The model under review builds one solid part; all positions refer to its coordinate system, in mm. A direction names the side the tool comes from. Round coordinates to 2 decimals unless told otherwise and drop trailing zeros. Order: outer loops, then holes, each group sorted by start corner. A loop starts at its lowest first (then second) coordinate and runs counter-clockwise, first axis right, second up. Notation, with made-up numbers: M 75.5,73 L 132.5,73 A25 cw 132.5,96 Z; hole C 1,56 d5. An arc over 180 degrees is marked long. Answer as CSV lines item,"result". Start each with the question number.
from build123d import *

# Parameters (mm, degrees)
SKETCH_1_W             = 45
SKETCH_1_H             = 38.5
EXTRUDE_1_DEPTH        = 60
SKETCH_2_R             = 15.1
CUT_EXTRUDE_1_DEPTH    = 50
SKETCH_3_R             = 2.5
EXTRUDE_2_DEPTH        = 5
SKETCH_4_R             = 1.5
CUT_EXTRUDE_2_DEPTH    = 78.620873481
PATTERN_LINEAR_1_COUNT = 2
PATTERN_LINEAR_1_PITCH = 20
FILLET_1_R             = 10


with BuildPart() as part:
    # 草圖1 → 填料-伸長1 (new body)
    with BuildSketch(Plane(origin=(0, 0, 0), x_dir=(1, 0, 0), z_dir=(0, 1, 0))):
        with Locations((-2.5, 0.75)):
            Rectangle(SKETCH_1_W, SKETCH_1_H)
    extrude(amount=EXTRUDE_1_DEPTH)

    # 草圖2 → 除料-伸長1 (cut)
    with BuildSketch(Plane(origin=(0, 60, 0), x_dir=(1, 0, 0), z_dir=(0, 1, 0))):
        with Locations(Location((0, 0, 0), (0, 0, 270))):
            Circle(SKETCH_2_R)
    extrude(amount=-CUT_EXTRUDE_1_DEPTH, mode=Mode.SUBTRACT)

    # 草圖3 → 填料-伸長2 (add)
    with BuildSketch(Plane.XY.offset(18.5)):
        Polygon((-25, 0), (-25, -15.5), (-5, -15.5), (20, 0), align=None)
        with Locations((-17.5, -8)):
            Circle(SKETCH_3_R, mode=Mode.SUBTRACT)
    extrude(amount=-EXTRUDE_2_DEPTH)

    # 草圖4 → 除料-伸長2 (cut, through all)
    with BuildSketch(Plane(origin=(20, 0, 0), x_dir=(0, 0, -1), z_dir=(1, 0, 0))):
        with Locations((0, 20)):
            Circle(SKETCH_4_R)
    cut_extrude_2 = extrude(amount=-CUT_EXTRUDE_2_DEPTH, mode=Mode.SUBTRACT)

    # 直線複製排列1: 除料-伸長2 ×2
    with Locations(*[(0, i * PATTERN_LINEAR_1_PITCH, 0) for i in range(1, PATTERN_LINEAR_1_COUNT)]):
        add(cut_extrude_2, mode=Mode.SUBTRACT)

    # 圓角1
    fillet_1_edges = [part.edges().sort_by_distance(p)[0] for p in [
        (-5, -15.5, 16),
        (-25, -15.5, 16),
    ]]
    fillet(fillet_1_edges, radius=FILLET_1_R)


solid = part.part
Item 1: Consider section B-B (z = 0). State the section outline as (x, y) points, and give its area (3 significant figures).
Item 2: Consider section A-A (y = 40). State the section outline as (x, z) points.
Item 3: Consider section D-D (x = -17.5). State the section outline as (y, z) points.
Item 4: Tool access review of faces 5 (the cylindrical face through (-14.74, 35.35, -3.27)), 6 (the cylindrical face through (-19.941, 38.536, 0.325)), 7 (the flat face through (-8, -6, 13.5)): name each direction out of +Z, -Z, +X, -X, +Y, -Y from which nothing blocks a thin tool from reaching the whole face with its end or side.
Item 5: Wall thickness on probe 1 along Y at (x, z) = (18.9, 0); probe 2 along Z at (x, y) = (18, 40); probe 3 along Y at (x, z) = (-17.5, -1): over which ranges is each line inside the solid? List them lowest first. Write a range as [from, to].
Item 6: For pin 1 (8 mm diameter, centred on x = 1.5, y = -5.5, fed in from -Z); pin 2 (1 mm diameter, centred on x = 6, z = 12.5, fed in from -Y); pin 3 (15 mm diameter, centred on x = 5.5, z = 4.5, fed in from +Y), all flat-tipped, find the tip position at first contact; note any pin that passes through.
Item 7: The part is to be moulded in two halves that separate along Y. For faces 1 (the cylindrical face through (17.546, 21.487, 0.195)), 2 (the flat face through (0, 10, 0)), 3 (the flat face through (-3, 0, -3)), 4 (the flat face through (-3, 23, 18.5)), say which applies: +Y half, -Y half, draft (parallel to the pull), parting line (faces both ways), or undercut.
Item 8: Consider section C-C (x = 0). State the section outline as (y, z) points.
Reported:
1,outline,"M -25,0 L 20,0 L 20,18.5 L 15.1,18.5 L 15.1,10 L -15.1,10 L -15.1,18.5 L -25,18.5 Z; M -25,21.5 L -15.1,21.5 L -15.1,38.5 L -25,38.5 Z; M -25,41.5 L -15.1,41.5 L -15.1,60 L -25,60 Z; M 15.1,21.5 L 20,21.5 L 20,38.5 L 15.1,38.5 Z; M 15.1,41.5 L 20,41.5 L 20,60 L 15.1,60 Z"
1,area,"1,100 mm²"
2,outline,"M -25,-20 L 20,-20 L 20,-1.5 L 15.03,-1.5 A15.1 cw -15.03,-1.5 L -25,-1.5 Z; M -25,1.5 L -15.03,1.5 A15.1 cw 15.03,1.5 L 20,1.5 L 20,18.5 L -25,18.5 Z"
3,outline,"M -15.18,13.5 L -10.5,13.5 L -10.5,18.5 L -15.18,18.5 Z; M -5.5,13.5 L 0,13.5 L 0,-20 L 60,-20 L 60,18.5 L -5.5,18.5 Z; hole C 20,0 d3; hole C 40,0 d3"
4,face 5,"+Y"
4,face 6,"+X, -X"
4,face 7,"-Z, +X, -X, -Y"
5,probe 1,"y = [0, 18.5], [21.5, 38.5], [41.5, 60]"
5,probe 2,"z = [-20, -1.5], [1.5, 18.5]"
5,probe 3,"y = [0, 18.88], [21.12, 38.88], [41.12, 60]"
6,pin 1,"stops at z = 13.5"
6,pin 2,"stops at y = 0"
6,pin 3,"stops at y = 10"
7,face 1,"undercut"
7,face 2,"+Y half"
7,face 3,"-Y half"
7,face 4,"draft"
8,outline,"M -12.4,13.5 L 0,13.5 L 0,-20 L 60,-20 L 60,-15.1 L 10,-15.1 L 10,15.1 L 60,15.1 L 60,18.5 L -12.4,18.5 Z"
